```python
from build123d import *

# Parameters (mm, degrees)
SKETCH1_R                 = 7
BOSS_EXTRUDE1_DEPTH       = 23
SKETCH3_W                 = 3
SKETCH3_H                 = 3
CUT_EXTRUDE1_DEPTH        = 21
SKETCH6_R                 = 8.5
BOSS_EXTRUDE2_DEPTH       = 28
SKETCH7_R                 = 9
BOSS_EXTRUDE3_DEPTH       = 2
M6X1_0_TAPPED_HOLE1_D     = 5
M6X1_0_TAPPED_HOLE1_DEPTH = 20
M6X1_0_TAPPED_HOLE1_TIP   = 1.502151548


with BuildPart() as part:
    # Sketch1 → Boss-Extrude1 (new body)
    with BuildSketch(Plane.XY):
        Circle(SKETCH1_R)
    extrude(amount=BOSS_EXTRUDE1_DEPTH)

    # Sketch3 → Cut-Extrude1 (cut)
    with BuildSketch(Plane(origin=(0, 0, 0), x_dir=(-1, 0, 0), z_dir=(0, 0, -1))):
        with Locations((0, 7)):
            Rectangle(SKETCH3_W, SKETCH3_H)
    extrude(amount=-CUT_EXTRUDE1_DEPTH, mode=Mode.SUBTRACT)

    # Sketch6 → Boss-Extrude2 (add)
    with BuildSketch(Plane.XY.offset(23)):
        Circle(SKETCH6_R)
    extrude(amount=BOSS_EXTRUDE2_DEPTH)

    # Sketch7 → Boss-Extrude3 (add)
    with BuildSketch(Plane(origin=(0, 0, 47), x_dir=(-1, 0, 0), z_dir=(0, 0, -1))):
        Circle(SKETCH7_R)
    extrude(amount=-BOSS_EXTRUDE3_DEPTH)

    # M6x1.0 Tapped Hole1
    with Locations(Plane.XY.offset(51)):
        with Locations((0, 0)):
            Hole(M6X1_0_TAPPED_HOLE1_D / 2, depth=M6X1_0_TAPPED_HOLE1_DEPTH)
            with Locations((0, 0, -(M6X1_0_TAPPED_HOLE1_DEPTH + M6X1_0_TAPPED_HOLE1_TIP / 2))):  # 118° drill point
                Cone(0, M6X1_0_TAPPED_HOLE1_D / 2, M6X1_0_TAPPED_HOLE1_TIP, mode=Mode.SUBTRACT)


solid = part.part
```
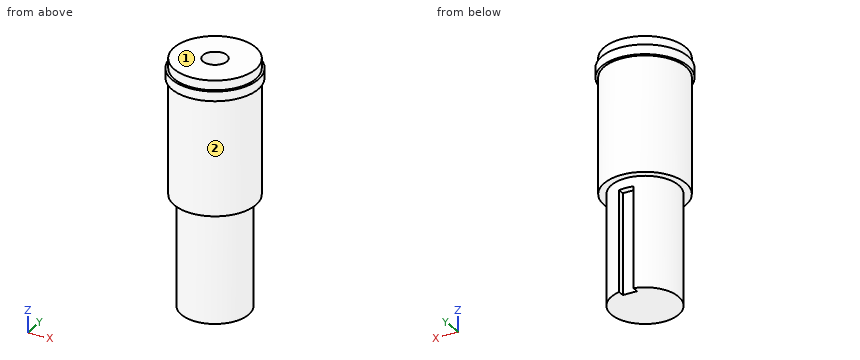
The listing builds one solid part. Answer for the finished solid, in the listing's coordinates (mm). Face numbers are marked on the shaded views. A direction names the side the tool comes from. Give positions to 0.01 mm unless a question says otherwise; leave off trailing zeros. Write each loop counter-clockwise with the first axis right and the second up, starting at its lowest first coordinate (ties: lowest second). Pieces come first, ordered by that corner, then holes. Notation, with made-up numbers: (70, 73) -> (104, 73) arc R12 ccw to (104, 92) -> close; hole circle Ø4 at (-3, 54.5). An arc over 180 degrees is marked (long way). Write item = value, one per line. Start each with the question number.
1) Each of these flat-tipped pins is pushed along its axis until it touches: pin 1 (10 mm diameter, centred on x = -7, z = 41, fed in from -Y); pin 2 (1 mm diameter, centred on y = -4.5, z = 35, fed in from -X); pin 3 (4 mm diameter, centred on x = 0, y = 0, fed in from -Z); pin 4 (1.2 mm diameter, centred on x = -0.5, y = 6.5, fed in from -Z). Where does it stop, or does it pass through?
2) The part is cut by section D-D, the plane x = -8. Determine the outline of the cut face in (y, z).
3) The part is cut by section B-B, the plane y = -5.25. Determine the outline of the cut face in (x, z).
4) Which of the six approach directions +Z, -Z, +X, -X, +Y, -Y give full straight-line access (tool end or side, diameter ignored) to the marked faces 1 and 2?
5) The part is cut by section A-A, the plane x = 6.5. Determine the outline of the cut face in (y, z), and give its area (3 significant figures).
6) The part is cut by section C-C, the plane z = 8. Determine the outline of the cut face in (x, y).
7) Straight lines are drawn through the part: line 1 along Y through (x, z) = (0, 43.75); line 2 along X through (y, z) = (0, 25). For each, find the intervals that lie inside material, in ascending order.
Solutions:
q1.pin_1 = -8.26
q1.pin_2 = -7.5
q1.pin_3 = 0
q1.pin_4 = 21
q2.outline = (-4.12, 47) -> (-2.87, 47) -> (-2.87, 23) -> (2.87, 23) -> (2.87, 47) -> (4.12, 47) -> (4.12, 49) -> (2.87, 49) -> (2.87, 51) -> (-2.87, 51) -> (-2.87, 49) -> (-4.12, 49) -> close
q3.outline = (-7.31, 47) -> (-6.68, 47) -> (-6.68, 23) -> (-4.63, 23) -> (-4.63, 0) -> (4.63, 0) -> (4.63, 23) -> (6.68, 23) -> (6.68, 47) -> (7.31, 47) -> (7.31, 49) -> (6.68, 49) -> (6.68, 51) -> (-6.68, 51) -> (-6.68, 49) -> (-7.31, 49) -> close
q4.face_1 = +Z, +X, -X, +Y, -Y
q4.face_2 = -Z
q5.outline = (-6.22, 47) -> (-5.48, 47) -> (-5.48, 23) -> (-2.6, 23) -> (-2.6, 0) -> (2.6, 0) -> (2.6, 23) -> (5.48, 23) -> (5.48, 47) -> (6.22, 47) -> (6.22, 49) -> (5.48, 49) -> (5.48, 51) -> (-5.48, 51) -> (-5.48, 49) -> (-6.22, 49) -> close
q5.area = 429 mm²
q6.outline = (-1.5, 5.5) -> (-1.5, 6.84) arc R7 ccw (long way) to (1.5, 6.84) -> (1.5, 5.5) -> close
q7.line_1 = -8.5 to -2.5, 2.5 to 8.5
q7.line_2 = -8.5 to 8.5
